```python
from build123d import *

# Parameters (mm, degrees)
F0_W     = 9
F0_H     = 15
F1_DEPTH = 20
F2_R     = 1.75
F3_DEPTH = 20.001
F4_R     = 3.5
F5_DEPTH = 5
F6_R     = 0.99999


# Not quite as in the source:
# - a fillet or chamfer is up to 0.001 mm smaller than in the source, because OpenCascade refuses the exact size


with BuildPart() as f1:
    # F0 (on Front) → F1 (new body)
    with BuildSketch(Plane.XZ):
        Rectangle(F0_W, F0_H)
    extrude(amount=F1_DEPTH)

    # F2 (on face) → F3 (cut, through all)
    with BuildSketch(Plane.XZ.offset(20)):
        Circle(F2_R)
    extrude(amount=-F3_DEPTH, mode=Mode.SUBTRACT)

    # F4 (on face) → F5 (cut)
    with BuildSketch(Plane.XZ.offset(20)):
        Circle(F4_R)
    extrude(amount=-F5_DEPTH, mode=Mode.SUBTRACT)

    # F6 (radius 1 in the source; OpenCascade refuses exactly that, so slightly less here)
    f6_edges = [f1.edges().sort_by_distance(p)[0] for p in [
        (4.5, -20, 0),
        (-4.5, -20, 0),
    ]]
    fillet(f6_edges, radius=F6_R)


solid = f1.part
```
Geometry check sheet. Reference: the model listing, model coordinates, mm. Round coordinates to 2 decimals unless told otherwise and drop trailing zeros. Order: outer loops, then holes, each group sorted by start corner. A loop starts at its lowest first (then second) coordinate and runs counter-clockwise, first axis right, second up. Notation, with made-up numbers: (24, -6) - (57, -6) arc R20 ccw to (57, 11) - close; hole circle Ø6 at (33.5, -39). An arc over 180 degrees is marked (long way). Use a Markdown table: item, result. Add a question column.
(1) Sectioned sample at C-C, the plane y = -16.75. Enter the section's corners in (x, z), and give its area (3 significant figures).
(2) Material ranges on line 1 along Z through (x, y) = (0, -17.3); line 2 along Z through (x, y) = (0, -5.5); line 3 along X through (y, z) = (-17.75, -0.75), recorded low to high. Write a range as [from, to].
(3) Sectioned sample at D-D, the plane z = -3.25. Enter the section's corners in (x, y), and give its area (3 significant figures).
(4) Release check for a two-part mould opening along Z. For faces 1 (the cylindrical face through (3.233, -17.535, -1.341)), 2 (the cylindrical face through (4.199, -19.715, 0.105)), 3 (the flat face through (0, -10, -7.5)), 4 (the flat face through (-2, -15, -1)) record: pulls with the +Z half, pulls with the -Z half, needs draft (parallel to the pull), parting line crosses it, or undercut.
(5) Sectioned sample at B-B, the plane x = 0. Enter the section's corners in (y, z).
Answers below:
| question | item | result |
|---|---|---|
| 1 | outline | (-4.5, -7.5) - (4.5, -7.5) - (4.5, 7.5) - (-4.5, 7.5) - close; hole circle Ø7 at (0, 0) |
| 1 | area | 96.5 mm² |
| 2 | line 1 | [-7.5, -3.5], [3.5, 7.5] |
| 2 | line 2 | [-7.5, -1.75], [1.75, 7.5] |
| 2 | line 3 | [-4.5, -3.42], [3.42, 4.5] |
| 3 | outline | (-4.5, -19) arc R1 ccw to (-3.5, -20) - (-1.3, -20) - (-1.3, -15) - (1.3, -15) - (1.3, -20) - (3.5, -20) arc R1 ccw to (4.5, -19) - (4.5, 0) - (-4.5, 0) - close |
| 3 | area | 167 mm² |
| 4 | face 1 | undercut |
| 4 | face 2 | needs draft |
| 4 | face 3 | pulls with the -Z half |
| 4 | face 4 | undercut |
| 5 | outline | (-20, -7.5) - (0, -7.5) - (0, -1.75) - (-15, -1.75) - (-15, -3.5) - (-20, -3.5) - close; (-20, 3.5) - (-15, 3.5) - (-15, 1.75) - (0, 1.75) - (0, 7.5) - (-20, 7.5) - close |
